```python
from build123d import *

# Parameters (mm, degrees)
SKETCH_1_W          = 4
SKETCH_1_H          = 0.6
EXTRUDE_1_DEPTH     = 2
SKETCH_1_3_W        = 0.6
SKETCH_1_3_H        = 2.5
EXTRUDE_2_DEPTH     = 1
SKETCH_1_4_R        = 3
EXTRUDE_3_DEPTH     = 7.5
CUT_EXTRUDE_1_DEPTH = 6.5


with BuildPart() as part:
    # 草图1 → 凸台-拉伸1 (new body)
    with BuildSketch(Plane(origin=(0, 0, 0), x_dir=(1, 0, 0), z_dir=(0, 1, 0))):
        Rectangle(SKETCH_1_W, SKETCH_1_H)
    extrude(amount=EXTRUDE_1_DEPTH)

    # 草图1<3> → 凸台-拉伸2 (add)
    with BuildSketch(Plane(origin=(0, 0, 0), x_dir=(1, 0, 0), z_dir=(0, 1, 0))):
        Rectangle(SKETCH_1_3_W, SKETCH_1_3_H)
    extrude(amount=EXTRUDE_2_DEPTH)

    # 草图1<4> → 凸台-拉伸3 (add)
    with BuildSketch(Plane(origin=(0, 0, 0), x_dir=(1, 0, 0), z_dir=(0, 1, 0))):
        with Locations(Location((0, 0, 0), (0, 0, 270))):
            Circle(SKETCH_1_4_R)
    extrude(amount=-EXTRUDE_3_DEPTH)

    # 草图2 → 切除-拉伸1 (cut)
    with BuildSketch(Plane.XZ.offset(7.5)):
        with BuildLine():
            ThreePointArc((-1.130029762, -2.230029762), (0, -2.5), (1.130029762, -2.230029762))
            Line((1.130029762, -2.230029762), (1.130029762, -1.130029762))
            Line((1.130029762, -1.130029762), (2.230029762, -1.130029762))
            ThreePointArc((2.230029762, -1.130029762), (2.5, 0), (2.230029762, 1.130029762))
            Line((2.230029762, 1.130029762), (1.130029762, 1.130029762))
            Line((1.130029762, 1.130029762), (1.130029762, 2.230029762))
            ThreePointArc((1.130029762, 2.230029762), (0, 2.5), (-1.130029762, 2.230029762))
            Line((-1.130029762, 2.230029762), (-1.130029762, 1.130029762))
            Line((-1.130029762, 1.130029762), (-2.230029762, 1.130029762))
            ThreePointArc((-2.230029762, 1.130029762), (-2.5, 0), (-2.230029762, -1.130029762))
            Line((-2.230029762, -1.130029762), (-1.130029762, -1.130029762))
            Line((-1.130029762, -1.130029762), (-1.130029762, -2.230029762))
        make_face()
    extrude(amount=-CUT_EXTRUDE_1_DEPTH, mode=Mode.SUBTRACT)


solid = part.part
```
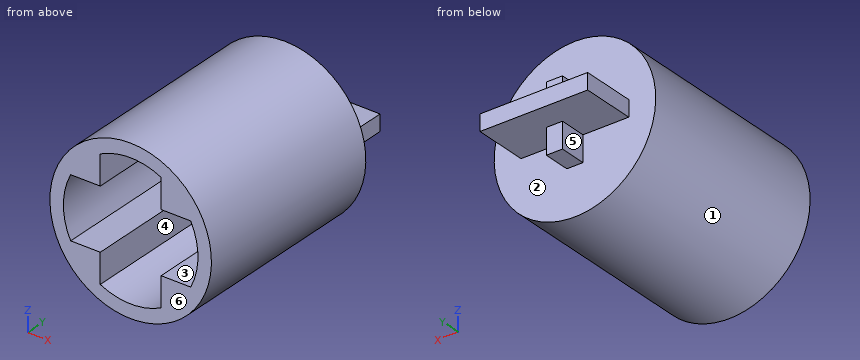
Could you check a few things on this model? Use its own coordinates, in mm. Face numbers are marked on the shaded views. A direction names the side the tool comes from. Coordinates: 2 decimals unless noted, no trailing zeros. Order: outer loops, then holes, each group sorted by start corner. A loop starts at its lowest first (then second) coordinate and runs counter-clockwise, first axis right, second up. Notation, with made-up numbers: M -33.75,14 L -10.75,14 A12 cw -10.75,37 Z; hole C 26,-2 d7. An arc over 180 degrees is marked long. Use one line per item in the form item = value. Start each with the question number.
1. We'd pull the mould along Z, two halves only. Please class the marked faces 1, 2 and 3: +Z half, -Z half, draft (parallel to the pull), parting line (faces both ways), or undercut.
2. Please list where these lines run through material, in increasing order: line 1 (Z direction, x = 0, y = 0.25); line 2 (Z direction, x = 0.15, y = -5.5); line 3 (Z direction, x = -1.85, y = -3.5).
3. On a 3-axis mill with a long thin cutter (end or side, diameter ignored), from which of +Z, -Z, +X, -X, +Y, -Y can I reach the whole of each face in a straight line? I mean the marked faces 4, 5 and 6. Say none if no direction works.
4. For pin 1 (2 mm diameter, centred on y = -5, z = -1.5, fed in from +X); pin 2 (1.2 mm diameter, centred on y = -3, z = -1.5, fed in from -X); pin 3 (0.9 mm diameter, centred on x = 1.5, y = -3, fed in from +Z), each with a flat end and sliding along its axis, tell me the tip position at first contact or that it passes through.
5. Suppose I cut it at D-D on y = -0.5. Write out the boundary of the cut face in (x, z), then the cut area to 3 significant figures.
6. Suppose I cut it at A-A on y = -4. Write out the boundary of the cut face in (x, z).
7. Suppose I cut it at C-C on z = 0. Write out the boundary of the cut face in (x, y).
8. Suppose I cut it at B-B on x = 0. Write out the boundary of the cut face in (y, z).
Geometry says:
q1.face_1 = parting line
q1.face_2 = draft
q1.face_3 = undercut
q2.line_1 = -1.25 to 1.25
q2.line_2 = -3 to -2.5, 2.5 to 3
q2.line_3 = -2.36 to -1.13, 1.13 to 2.36
q3.face_4 = -Y
q3.face_5 = -Z, -X, +Y
q3.face_6 = +Z, -Z, +X, -X, -Y
q4.pin_1 = 2.96
q4.pin_2 = -2.86
q4.pin_3 = 2.81
q5.outline = C 0,0 d6
q5.area = 28.3 mm^2
q6.outline = C 0,0 d6; hole M -2.23,-1.13 L -1.13,-1.13 L -1.13,-2.23 A2.5 ccw 1.13,-2.23 L 1.13,-1.13 L 2.23,-1.13 A2.5 ccw 2.23,1.13 L 1.13,1.13 L 1.13,2.23 A2.5 ccw -1.13,2.23 L -1.13,1.13 L -2.23,1.13 A2.5 ccw Z
q7.outline = M -3,-7.5 L -2.5,-7.5 L -2.5,-1 L 2.5,-1 L 2.5,-7.5 L 3,-7.5 L 3,0 L 2,0 L 2,2 L -2,2 L -2,0 L -3,0 Z
q8.outline = M -7.5,-3 L 0,-3 L 0,-1.25 L 1,-1.25 L 1,-0.3 L 2,-0.3 L 2,0.3 L 1,0.3 L 1,1.25 L 0,1.25 L 0,3 L -7.5,3 L -7.5,2.5 L -1,2.5 L -1,-2.5 L -7.5,-2.5 Z
